Source: CAD feature listing. Evaluate the final solid. Frame: model axes, mm. Coordinates: 2 decimals unless noted, no trailing zeros. Order: outer loops, then holes, each group sorted by start corner. A loop starts at its lowest first (then second) coordinate and runs counter-clockwise, first axis right, second up.
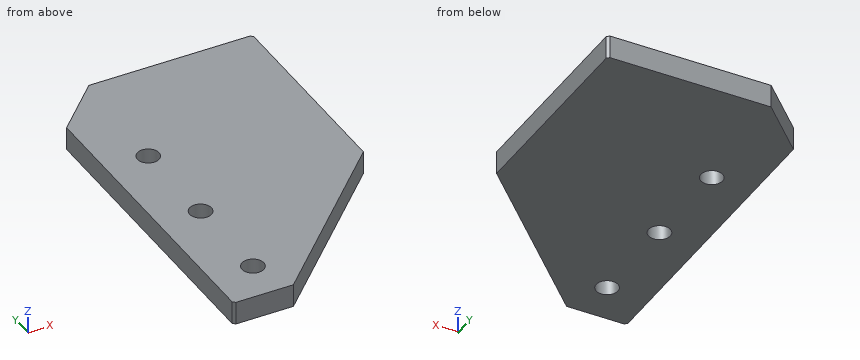
```python
from build123d import *

# Parameters (mm, degrees)
BOSS_EXTRUDE1_DEPTH  = 4.7625
M8_CLEARANCE_HOLE1_D = 9
CHAMFER1_SIZE        = 1


with BuildPart() as part:
    # Sketch1 → Boss-Extrude1 (new, symmetric)
    with BuildSketch(Plane.XY):
        Polygon((-72.5, -37.5), (-47.751262658, -37.5), (15, 25.251262658), (15, 110), (-52.5, 110), (-72.5, 90), align=None)
    extrude(amount=BOSS_EXTRUDE1_DEPTH, both=True)

    # M8 Clearance Hole1 (through all)
    with Locations(Plane.XY.offset(4.7625)):
        with Locations((-55, 60), (-55, 20), (-55, -20)):
            Hole(M8_CLEARANCE_HOLE1_D / 2)

    # Chamfer1
    chamfer1_edges = [part.edges().sort_by_distance(p)[0] for p in [
        (15, 110, 0),
        (-72.5, -37.5, 0),
    ]]
    chamfer(chamfer1_edges, length=CHAMFER1_SIZE)


solid = part.part
```
1. Ray query, line 1 (Y direction, x = -53, z = -3.75); line 2 (Y direction, x = -59, z = 1.5); line 3 (X direction, y = 17.5, z = 4). Return the intervals inside material, ascending.
Findings:
line 1: y = -37.5 to -24.03, -15.97 to 15.97, 24.03 to 55.97, 64.03 to 109.5
line 2: y = -37.5 to -22.06, -17.94 to 17.94, 22.06 to 57.94, 62.06 to 103.5
line 3: x = -72.5 to -58.74, -51.26 to 7.25
2. Section query A-A on x = -55. Return loops of the section in (y, z), plus the area to 3 significant figures.
Findings:
outline: (-37.5, -4.76) - (-24.5, -4.76) - (-24.5, 4.76) - (-37.5, 4.76) - close; (-15.5, -4.76) - (15.5, -4.76) - (15.5, 4.76) - (-15.5, 4.76) - close; (24.5, -4.76) - (55.5, -4.76) - (55.5, 4.76) - (24.5, 4.76) - close; (64.5, -4.76) - (107.5, -4.76) - (107.5, 4.76) - (64.5, 4.76) - close
area: 1,120 mm2
3. Section query B-B on z = 0.25. Return loops of the section in (x, y).
Findings:
outline: (-72.5, -36.5) - (-71.5, -37.5) - (-47.75, -37.5) - (15, 25.25) - (15, 109) - (14, 110) - (-52.5, 110) - (-72.5, 90) - close; hole circle Ø9 at (-55, -20); hole circle Ø9 at (-55, 20); hole circle Ø9 at (-55, 60)
4. Section query D-D on y = 20. Return loops of the section in (x, z), plus the area to 3 significant figures.
Findings:
outline: (-72.5, -4.76) - (-59.5, -4.76) - (-59.5, 4.76) - (-72.5, 4.76) - close; (-50.5, -4.76) - (9.75, -4.76) - (9.75, 4.76) - (-50.5, 4.76) - close
area: 698 mm2
5. Pin query (flat end, axial travel): P1, Ø3, axis at x = -30, z = 1.5, coming from the -Y side; P2, Ø7, axis at x = -55, y = 60, coming from the +Z side; P3, Ø2, axis at x = -33.5, z = 0, coming from the -Y side. Return the tip coordinate at first contact, or that it passes through.
Findings:
P1: stops at y = -21.25
P2: passes through
P3: stops at y = -24.25
6. Section query C-C on y = 60. Return loops of the section in (x, z), plus the area to 3 significant figures.
Findings:
outline: (-72.5, -4.76) - (-59.5, -4.76) - (-59.5, 4.76) - (-72.5, 4.76) - close; (-50.5, -4.76) - (15, -4.76) - (15, 4.76) - (-50.5, 4.76) - close
area: 748 mm2
